Part model, mm, in its own coordinate system. A direction names the side the tool comes from. Give positions to 0.01 mm unless a question says otherwise; leave off trailing zeros. Order: outer loops, then holes, each group sorted by start corner. A loop starts at its lowest first (then second) coordinate and runs counter-clockwise, first axis right, second up. Notation, with made-up numbers: M 44,63 L 64,63 A18 cw 64,94 Z; hole C 48,88.25 d10. An arc over 180 degrees is marked long. Answer as a JSON object with one key per item and string values.
from build123d import *

# Parameters (mm, degrees)
F0_W     = 90
F0_H     = 80
F1_DEPTH = 1.5
F3_DEPTH = 25
F4_D     = 5.2
F4_DEPTH = 5
F4_TIP   = 1.5622376095
F5_SIZE  = 1.2


with BuildPart() as f1:
    # F0 (on Top) → F1 (new body)
    with BuildSketch(Plane.XY):
        with Locations((4.5240691602, -8.1039099395)):
            Rectangle(F0_W, F0_H)
    extrude(amount=F1_DEPTH)

    # F2 (on face) → F3 (join)
    with BuildSketch(Plane.XY.offset(1.5)):
        Polygon((0, 31.8960900605), (-13.9759308398, 31.8960900605), (-13.9759308398, 18.8960900605), (-40.4759308398, 18.8960900605), (-40.4759308398, -35.1039099395), (-13.9759308398, -35.1039099395), (-13.9759308398, -48.1039099395), (23.0240691602, -48.1039099395), (23.0240691602, -35.1039099395), (49.5240691602, -35.1039099395), (49.5240691602, 18.8960900605), (23.0240691602, 18.8960900605), (23.0240691602, 31.8960900605), align=None)
    extrude(amount=F3_DEPTH)

    # F4
    with Locations(Plane.XY.offset(1.5)):
        with Locations((-21.9759307802, 25.3960900605), (31.0240691602, 25.3960900605), (31.0240691602, -41.6039099395), (-21.9759307802, -41.6039099395)):
            Hole(F4_D / 2, depth=F4_DEPTH)
            with Locations((0, 0, -(F4_DEPTH + F4_TIP / 2))):  # 118° drill point
                Cone(0, F4_D / 2, F4_TIP, mode=Mode.SUBTRACT)

    # F5
    f5_edges = [f1.edges().sort_by_distance(p)[0] for p in [
        (-40.475931, -8.10391, 26.5),
        (-13.975931, -41.60391, 26.5),
        (-13.975931, 25.39609, 26.5),
        (23.024069, 25.39609, 26.5),
        (23.024069, -41.60391, 26.5),
        (49.524069, -8.10391, 26.5),
    ]]
    chamfer(f5_edges, length=F5_SIZE)


solid = f1.part
1. Which spindle directions (+Z, -Z, +X, -X, +Y, -Y) get a long thin tool onto all of the face, cutting with end or side? Do faces 4 (the flat face through (-40.476, -9, 12)), 5 (the flat face through (-26, 18.896, 14)), 6 (the flat face through (23.024, -42, 13)), 7 (the flat face through (36, 18.896, 14)), 8 (the flat face through (-27, -35.104, 14)). Say none if no direction does.
Worked answers:
{"face 4": "+Z, -Z, -X, +Y, -Y", "face 5": "+Z, -X, +Y", "face 6": "+Z, +X, -Y", "face 7": "+Z, +X, +Y", "face 8": "+Z, -X, -Y"}
2. Cut at A-A on z = 15.75. Give the cut face in (x, y).
Worked answers:
{"outline": "M -40.48,-35.1 L -13.98,-35.1 L -13.98,-48.1 L 23.02,-48.1 L 23.02,-35.1 L 49.52,-35.1 L 49.52,18.9 L 23.02,18.9 L 23.02,31.9 L -13.98,31.9 L -13.98,18.9 L -40.48,18.9 Z"}
3. Cut at B-B on x = -33.5. Give the cut face in (y, z).
Worked answers:
{"outline": "M -48.1,0 L 31.9,0 L 31.9,1.5 L 18.9,1.5 L 18.9,26.5 L -35.1,26.5 L -35.1,1.5 L -48.1,1.5 Z"}
4. Two-plate mould, pull along Y, no slides. Class faces 1 (the cylindrical face through (31.363, 27.974, 0.739)), 2 (the flat face through (35, -35.104, 14)), 3 (the flat face through (36, 25, 1.5)): +Y half, -Y half, draft (parallel to the pull), parting line (faces both ways), or undercut.
Worked answers:
{"face 1": "undercut", "face 2": "-Y half", "face 3": "draft"}
5. Pin check, flat tips, straight feed: P1, Ø4, axis at y = 25, z = 13, coming from the +X side; P2, Ø8.5, axis at x = -21.98, y = -41.6, coming from the +Z side; P3, Ø12.5, axis at x = -30.5, z = 19.5, coming from the +Y side. Stop position of each tip, or through.
Worked answers:
{"P1": "stops at x = 23.02", "P2": "stops at z = 1.5", "P3": "stops at y = 18.9"}
6. Probe line 1 along Y through (x, z) = (-35, 4.75); line 2 along X through (y, z) = (23.5, 20); line 3 along Z through (x, y) = (-16, 23). List the from-to ranges inside material, lowest first.
Worked answers:
{"line 1": "y = -35.1 to 18.9", "line 2": "x = -13.98 to 23.02", "line 3": "z = 0 to 1.5"}
